from build123d import *

# Parameters (mm, degrees)
SKETCH1_W          = 40
SKETCH1_H          = 43.18
BASE_DEPTH         = 2.4638
SKETCH2_W          = 12.7
SKETCH2_H          = 2.4638
BOTTOM_TABS_DEPTH  = 5.334
SKETCH3_R          = 6.875
SKETCH3_W          = 5.261651729
SKETCH3_H          = 1.351567934
SKETCH3_W_2        = 4.974619722
MOUNT_POINTS_DEPTH = 59.911651737
SKETCH4_R          = 4.245
CUT_EXTRUDE2_DEPTH = 36.250138525


with BuildPart() as part:
    # Sketch1 → Base (new body)
    with BuildSketch(Plane.XY):
        with Locations((20, 21.59)):
            Rectangle(SKETCH1_W, SKETCH1_H)
    extrude(amount=BASE_DEPTH)

    # Sketch2 → Bottom Tabs (add)
    with BuildSketch(Plane.XZ):
        with Locations((6.35, 1.2319)):
            Rectangle(SKETCH2_W, SKETCH2_H)
        with Locations((33.65, 1.2319)):
            Rectangle(SKETCH2_W, SKETCH2_H)
    extrude(amount=BOTTOM_TABS_DEPTH)

    # Sketch3 → Mount Points (cut, through all)
    with BuildSketch(Plane.XY.offset(2.4638)):
        with Locations((20, 21.59)):
            Circle(SKETCH3_R)
        with Locations((32.854435388, 21.59)):
            Rectangle(SKETCH3_W, SKETCH3_H)
        with Locations((4.5, 21.59)):
            Rectangle(SKETCH3_W_2, SKETCH3_H)
    extrude(amount=-MOUNT_POINTS_DEPTH, mode=Mode.SUBTRACT)

    # Sketch4 → Cut-Extrude2 (cut, through all)
    with BuildSketch(Plane(origin=(18.246403628, 22.293576812, 2.4638), x_dir=(1, 0, 0), z_dir=(0, 0, 1))):
        with Locations((15.813596372, 23.649057543)):
            Circle(SKETCH4_R)
    extrude(amount=-CUT_EXTRUDE2_DEPTH, mode=Mode.SUBTRACT)


solid = part.part
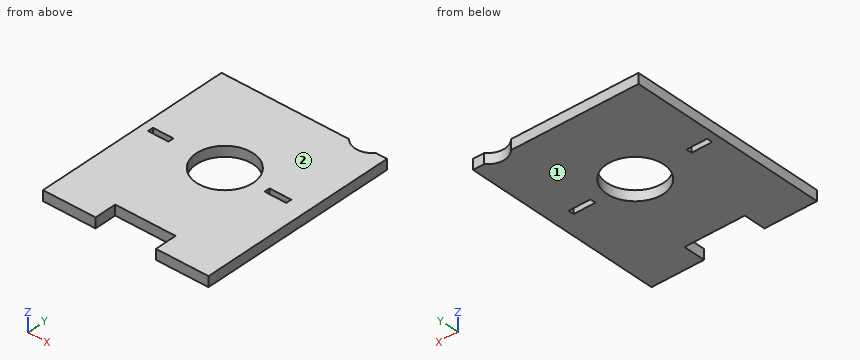
For this review, take the finished solid that the model builds, in its own axes (mm). Face numbers are marked on the shaded views. Round coordinates to 2 decimals unless told otherwise and drop trailing zeros. Loops run counter-clockwise (first coordinate to the right, second up) from the corner with the lowest first, then second, coordinate; pieces in that order, holes last. Notation, with made-up numbers: (58.25, 46) - (88.25, 46) arc R19 ccw to (88.25, 65) - close; hole circle Ø9 at (18.25, 9.5). An arc over 180 degrees is marked (long way). Use one line per item in the form item = value.
Item 1: Consider section A-A on x = 20. Write out the cut boundary in (y, z) (3 decimals), then the cut area to 3 significant figures.
Answers:
outline = (0, 0) - (14.715, 0) - (14.715, 2.464) - (0, 2.464) - close; (28.465, 0) - (43.18, 0) - (43.18, 2.464) - (28.465, 2.464) - close
area = 72.5 mm^2
Item 2: Consider section B-B on y = 21.59. Write out the cut boundary in (x, z) (3 decimals).
Answers:
outline = (0, 0) - (2.013, 0) - (2.013, 2.464) - (0, 2.464) - close; (6.987, 0) - (13.125, 0) - (13.125, 2.464) - (6.987, 2.464) - close; (26.875, 0) - (30.224, 0) - (30.224, 2.464) - (26.875, 2.464) - close; (35.485, 0) - (40, 0) - (40, 2.464) - (35.485, 2.464) - close
Item 3: Mouldability with a two-part tool opening along Z and no side actions: class the marked faces 1 and 2 as +Z half, -Z half, draft (parallel to the pull), parting line (faces both ways), or undercut.
Answers:
face_1 = -Z half
face_2 = +Z half
Item 4: Consider section D-D on x = 33. Write out the cut boundary in (y, z).
Answers:
outline = (-5.33, 0) - (20.91, 0) - (20.91, 2.46) - (-5.33, 2.46) - close; (22.27, 0) - (41.83, 0) - (41.83, 2.46) - (22.27, 2.46) - close
Item 5: Consider section C-C on z = 0.4. Write out the cut boundary in (x, y) (3 decimals).
Answers:
outline = (0, -5.334) - (12.7, -5.334) - (12.7, 0) - (27.3, 0) - (27.3, -5.334) - (40, -5.334) - (40, 43.18) - (37.283, 43.18) arc R4.245 cw to (30.837, 43.18) - (0, 43.18) - close; hole (2.013, 20.914) - (6.987, 20.914) - (6.987, 22.266) - (2.013, 22.266) - close; hole circle Ø13.75 at (20, 21.59); hole (30.224, 20.914) - (35.485, 20.914) - (35.485, 22.266) - (30.224, 22.266) - close
Item 6: Clearance check with flat-ended pins moving along their axes: P1, Ø1.2, axis at x = 20, z = 1.5, coming from the -Y side; P2, Ø8, axis at x = 8.5, y = 12.5, coming from the -Z side; P3, Ø1.2, axis at x = 32.5, z = 1.5, coming from the +Y side. State where each tip first meets the part, or that it passes through.
Answers:
P1 = 0
P2 = 0
P3 = 42.29
Item 7: For line 1 (Y direction, x = 20, z = 0.7) (3 decimals); line 2 (Y direction, x = 30.5, z = 2.25); line 3 (X direction, y = 27.5, z = 1.2), list the stretches that pass through material, from the lowest coordinate up.
Answers:
line_1 = 0 to 14.715, 28.465 to 43.18
line_2 = -5.33 to 20.91, 22.27 to 43.18
line_3 = 0 to 16.49, 23.51 to 40
